Autodesk Inventor part; units mm, degrees
ref_plane "YZ Plane" through (0, 0, 0) normal (1, 0, 0) x (0, 1, 0)
ref_plane "XZ Plane" through (0, 0, 0) normal (0, 1, 0) x (-1, 0, 0)
ref_plane "XY Plane" through (0, 0, 0) normal (0, 0, 1) x (1, 0, 0)
sketch "Sketch1" plane through (0, 0, 0) normal (0, 1, 0) x (-1, 0, 0)
  arc A0 (0, -5) -> (0, 5) centre (0, 0) ccw
  line L0 (0, 5) -> (0, -5)
  dimension "d0" = 10
extrude "Extrusion1" add sketch "Sketch1" along normal blind 10
sketch "Sketch2" plane through (0, 0, 0) normal (1, 0, 0) x (0, 1, 0)
  line L0 (8.0172, -4.5) -> (8.0172, 4.5)
  line L1 (8.0172, 4.5) -> (2.5172, 4.5)
  line L2 (2.5172, -4.5) -> (0.0172, -2)
  line L3 (2.5172, 4.5) -> (0.0172, 2)
  line L4 (0.0172, -2) -> (0.0172, 2)
  line L5 (8.0172, -4.5) -> (2.5172, -4.5)
  point P0 (0, 0)
  dimension "d3" = 9
  dimension "d4" = 8
sketch "Sketch3" plane through (0, 0, 0) normal (1, 0, 0) x (0, 1, 0)
  line L0 (0, 2) -> (3, 5)
  arc A0 (3, 5) -> (0, 2) centre (1, 4) ccw
  line L1 (0, -2) -> (4, -6)
  arc A1 (0, -2) -> (4, -6) centre (1.75, -4.25) ccw
  line L2 (8.0325, 5) -> (11, 5)
  line L3 (11, 5) -> (11, -6)
  line L4 (11, -6) -> (8.0325, -6)
  line L5 (8.0325, -6) -> (8.0325, 5)
  line L6 (2.4911, 4.4911) -> (5, 7)
  line L7 (2.4911, 4.4911) -> (8.0325, 4.4911)
  arc A2 (8.0325, 4.4911) -> (5, 7) centre (7, 6.3303) ccw
  line L8 (2.4911, -4.4911) -> (8.5706, -4.4911)
  arc A3 (2.4911, -4.4911) -> (8.5706, -4.4911) centre (5.5309, -7.5041) ccw
  point P0 (0, 0)
extrude "Extrusion2" cut sketch "Sketch3" against normal through all
sketch "Sketch4" plane through (0, 0, 0) normal (0, 1, 0) x (-1, 0, 0)
  arc A0 (1.0726, -4.4911) -> (1.0726, 4.4911) centre (-1.125, 0) ccw
  arc A1 (1.0726, 4.4911) -> (1.0726, -4.4911) centre (-0.4517, 0) ccw
  point P0 (0, 0)
  point P1 (2.1976, -4.4911)
  point P2 (2.1976, 4.4911)
  dimension "d9" = 1.125
  dimension "d10" = 1.125
extrude "Extrusion3" cut sketch "Sketch4" along normal through all both and the other way through all
sketch "Sketch5" plane through (0, 0, 0) normal (1, 0, 0) x (0, 1, 0)
  line L0 (0.88, -1.6179) -> (0.88, 1.5021)
  line L1 (7.1622, 3.4985) -> (2.8462, 3.4985)
  line L2 (7.1622, -3.4985) -> (7.1622, 3.4985)
  line L3 (7.1622, -3.4985) -> (2.8462, -3.4985)
  line L4 (0, 2) -> (0, -2)
  line L5 (8.0325, 4.4911) -> (8.0325, -4.4911)
  line L6 (0, 2) -> (2.4911, 4.4911)
  line L7 (2.4911, 4.4911) -> (8.0325, 4.4911)
  line L8 (8.0325, 4.4911) -> (8.0325, -4.4911)
  line L9 (8.0325, -4.4911) -> (2.4911, -4.4911)
  line L10 (2.4911, -4.4911) -> (0, -2)
  line L11 (0, 2) -> (0, -2)
  line L12 (0.88, 1.5021) -> (2.8462, 3.4985)
  line L13 (0.88, -1.6179) -> (2.8462, -3.4985)
  line L14 (0.88, 6.0552) -> (0.88, -6.997)
  arc A0 (0.88, 6.0552) -> (0.88, -6.997) centre (3.0168, -0.4709) ccw
  line L15 (0.88, 1.5021) -> (5.9184, 6.6178)
  line L16 (0.88, 1.5021) -> (0.88, 9.8799)
  arc A1 (5.9184, 6.6178) -> (0.88, 9.8799) centre (3.8488, 8.9433) ccw
  line L17 (2.8462, 3.4985) -> (14.9244, 3.4985)
  line L18 (2.8462, 3.4985) -> (9.8914, 10.6517)
  arc A2 (14.9244, 3.4985) -> (9.8914, 10.6517) centre (9.6254, 5.1173) ccw
  line L19 (7.1622, 3.4985) -> (16.5233, 3.4985)
  line L20 (7.1622, 3.4985) -> (7.1622, -12.1727)
  arc A3 (7.1622, -12.1727) -> (16.5233, 3.4985) centre (7.081, -1.4927) ccw
  line L21 (7.1622, -3.4985) -> (7.1622, -15.0508)
  line L22 (7.1622, -3.4985) -> (2.8462, -3.4985)
  line L23 (2.8462, -3.4985) -> (3.0168, -16.7137)
  arc A4 (3.0168, -16.7137) -> (7.1622, -12.1727) centre (6.096, -15.362) ccw
  line L24 (0.88, -1.6179) -> (0.88, -10.6889)
  line L25 (0.88, -1.6179) -> (2.8462, -3.4985)
  line L26 (2.8462, -3.4985) -> (2.953, -11.7746)
  arc A5 (0.88, -10.6889) -> (2.953, -11.7746) centre (2.2295, -10.6341) ccw
  point P0 (0, 0)
  dimension "d16" = 0.88
  dimension "d18" = 0.8703
  dimension "d21" = 0.9927
  dimension "d23" = 0.9927
  dimension "d24" = 3.12
  dimension "d26" = 4.316
  dimension "d27" = 4.316
extrude "Extrusion4" cut sketch "Sketch5" against normal through all contours L14 L10 L4 L6 L0 | L13 L23 L9 L10 L14 | L14 L6 L7 L15 L12 | L3 L20 L9 L23 | L14 A0 L6 L4 L10 | L10 L9 L23 A5 L24 L14 | L15 L7 L5 L17 L1 | L14 L16 A1 L18 L15 L7 L6 | L2 L17 L5 L9 L20 | L9 L20 A4 L23 | L15 A1 L18 A2 L17 L5 L7 | L9 L5 L17 L19 A3 L20 | L18 A1
sketch "Sketch6" plane through (0, 0, 0) normal (1, 0, 0) x (0, 1, 0)
  circle A0 centre (3.28, -0.3734) radius 1.575
  line L0 (0.88, -1.6179) -> (0.88, 1.5021)
  point P0 (0, 0)
  dimension "d31" = 3.15
  dimension "d32" = 2.4
extrude "Extrusion5" add sketch "Sketch6" against normal blind 15
sketch "Sketch7" plane through (0, 0, 0) normal (0, 1, 0) x (-1, 0, 0)
  arc A0 (2.4472, -3.4985) -> (3.606, -1.6179) centre (-1.125, 0) ccw
  arc A1 (3.644, 1.5021) -> (2.4472, 3.4985) centre (-1.125, 0) ccw
  arc A2 (3.606, -1.6179) -> (3.644, 1.5021) centre (-1.125, 0) ccw
  arc A3 (2.4472, 3.4985) -> (2.4472, -3.4985) centre (2.4472, 0) ccw
  point P0 (0, 0)
extrude "Extrusion6" cut sketch "Sketch7" along normal through all
sketch "Sketch8" plane through (-15, 3.28, -0.3734) normal (-1, 0, 0) x (0, 0, 1)
  circle A0 centre (0, 0) radius 0.5375
  point P0 (0.3734, -3.28)
  dimension "d37" = 1.075
extrude "Extrusion7" cut sketch "Sketch8" against normal blind 10
properties part number "10mm_radius_labmaker_cSkull_mold_window_stabilizer_surface_bigger_May1519"
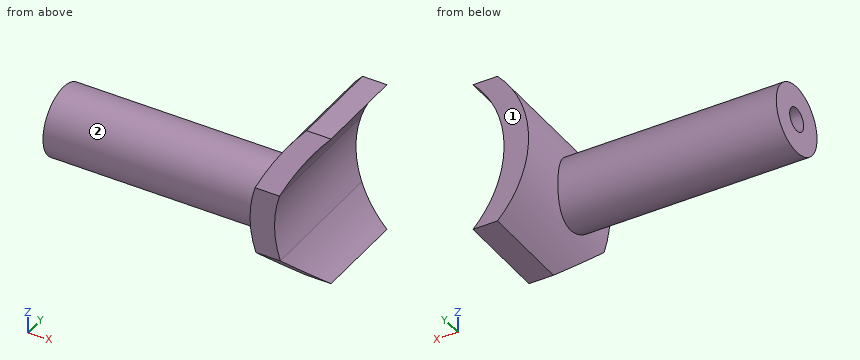
Design review of the part built by this model. Coordinates are the model's own, in mm. Face numbers are marked on the shaded views. A direction names the side the tool comes from. Coordinates: 2 decimals unless noted, no trailing zeros. Loops run counter-clockwise (first coordinate to the right, second up) from the corner with the lowest first, then second, coordinate; pieces in that order, holes last. Notation, with made-up numbers: (-4.5, 58.25) - (35.5, 58.25) arc R24 cw to (35.5, 93.25) - close; hole circle Ø6 at (46.25, 51.5). An arc over 180 degrees is marked (long way). Use CSV: the item, a comma, the result in double quotes. Start each with the question number.
1. For the marked faces 1 and 2, list the 3-axis set-ups (+Z, -Z, +X, -X, +Y, -Y) from which the entire face can be reached by the end or side of a thin tool; tool diameter is ignored.
2. Add section D-D on y = 6.25. Give the boundary of the cut face in (x, z).
3. Add section B-B on z = 0.75. Give the boundary of the cut face in (x, y), plus the area to 3 significant figures.
4. Clearance check with flat-ended pins moving along their axes: pin 1 (1.4 mm diameter, centred on y = 3.28, z = -0.37, fed in from +X); pin 2 (3 mm diameter, centred on x = -10, z = 2.5, fed in from +Y); pin 3 (3 mm diameter, centred on x = -5.5, y = 3, fed in from -Z). State where each tip first meets the part, or that it passes through.
5. Add section A-A on y = 3.28. Give the boundary of the cut face in (x, z).
6. To check wall thickness, follow probe 1 along X at (y, z) = (3.5, 1.5); probe 2 along X at (y, z) = (4.75, 0) (3 decimals); probe 3 along Y at (x, z) = (-11.25, 0). State the ranges of each line that lie inside material, in increasing order.
Resolved:
1,face 1,"+Z, -Z, +X, -X, +Y"
1,face 2,"-X"
2,outline,"(-3.64, 1.5) arc R5 cw to (-2.45, 3.5) - (-3.57, 3.5) arc R5 ccw to (-3.57, -3.5) - (-2.45, -3.5) arc R5 cw to (-3.61, -1.62) arc R5 cw to start"
3,outline,"(-15, 2.18) - (-4.94, 2.18) - (-4.94, 0.88) - (-3.82, 0.88) - (-3.82, 7.16) - (-4.94, 7.16) - (-4.94, 4.38) - (-15, 4.38) - close"
3,area,"29.3 mm2"
4,pin 1,"x = -3.76"
4,pin 2,"y = 4.05"
4,pin 3,"z = -3"
5,outline,"(-15, -1.95) - (-4.6, -1.95) arc R5 ccw to (-3.57, -3.5) - (-2.45, -3.5) arc R5 cw to (-3.61, -1.62) arc R5 cw to (-3.64, 1.5) arc R5 cw to (-2.45, 3.5) - (-3.57, 3.5) arc R5 ccw to (-4.85, 1.2) - (-15, 1.2) - (-15, 0.16) - (-5, 0.16) - (-5, -0.91) - (-15, -0.91) - close"
6,probe 1,"-4.77 to -3.64"
6,probe 2,"-15 to -3.875"
6,probe 3,"1.75 to 2.89, 3.67 to 4.81"
